from build123d import *

# Parameters (mm, degrees)
BOSS_EXTRUDE1_DEPTH = 8.89
SKETCH2_R           = 6.35
CUT_EXTRUDE1_DEPTH  = 27.197420728
SKETCH3_R           = 1.5
SKETCH3_R_2         = 1.45
BOSS_EXTRUDE2_DEPTH = 2.54


with BuildPart() as part:
    # Sketch1 → Boss-Extrude1 (new body)
    with BuildSketch(Plane.XY):
        with BuildLine():
            Line((-9.350252532, -14.130551756), (9.350252532, -14.130551756))
            Line((9.350252532, -14.130551756), (14.3, -9.180804288))
            Line((14.3, -9.180804288), (14.3, 12.34601478))
            ThreePointArc((14.3, 12.34601478), (0, 20.069448244), (-14.3, 12.34601478))
            Line((-14.3, 12.34601478), (-14.3, -9.180804288))
            Line((-14.3, -9.180804288), (-9.350252532, -14.130551756))
        make_face()
    extrude(amount=BOSS_EXTRUDE1_DEPTH)

    # Sketch2 → Cut-Extrude1 (cut, through all)
    with BuildSketch(Plane(origin=(0, 0, 0), x_dir=(-1, 0, 0), z_dir=(0, 0, -1))):
        with Locations((0, 5.99601478)):
            Circle(SKETCH2_R)
    extrude(amount=-CUT_EXTRUDE1_DEPTH, mode=Mode.SUBTRACT)

    # Sketch3 → Boss-Extrude2 (add)
    # profile 1 of 2: a face of its own
    with BuildSketch(Plane.XY.offset(8.89)):
        with BuildLine():
            Line((-14.3, 12.34601478), (-24.034198127, 9.287357095))
            ThreePointArc((-24.034198127, 9.287357095), (-26.45, 5.99601478), (-24.034198127, 2.704672465))
            Line((-24.034198127, 2.704672465), (-14.3, -0.35398522))
            Line((-14.3, -0.35398522), (-14.3, 12.34601478))
        make_face()
        with Locations((-16.2, 5.99601478)):
            Circle(SKETCH3_R, mode=Mode.SUBTRACT)
        with Locations((-23, 5.99601478)):
            Circle(SKETCH3_R_2, mode=Mode.SUBTRACT)
    # profile 2 of 2: a face of its own
    with BuildSketch(Plane.XY.offset(8.89)):
        with BuildLine():
            Line((14.3, 12.34601478), (14.3, -0.35398522))
            Line((14.3, -0.35398522), (24.034198127, 2.704672465))
            ThreePointArc((24.034198127, 2.704672465), (26.45, 5.99601478), (24.034198127, 9.287357095))
            Line((24.034198127, 9.287357095), (14.3, 12.34601478))
        make_face()
        with Locations((16.2, 5.99601478)):
            Circle(SKETCH3_R, mode=Mode.SUBTRACT)
        with Locations((23, 5.99601478)):
            Circle(SKETCH3_R_2, mode=Mode.SUBTRACT)
    extrude(amount=-BOSS_EXTRUDE2_DEPTH)


solid = part.part
Can you work these out from the model? Positions are in its coordinate system, mm. A direction names the side the tool comes from. Coordinates: 2 decimals unless noted, no trailing zeros. Loops run counter-clockwise (first coordinate to the right, second up) from the corner with the lowest first, then second, coordinate; pieces in that order, holes last. Notation, with made-up numbers: M 31.5,-39 L 83.5,-39 A21 cw 83.5,-11 Z; hole C 38.25,14.5 d9. An arc over 180 degrees is marked long. Return JSON: item names as keys, results as strings. Group by question number.
Item 1: Imagine slicing it at D-D (y = -1). Please give me the cut outline in (x, z), and give its area (3 significant figures).
Item 2: On a 3-axis mill with a long thin cutter (end or side, diameter ignored), from which of +Z, -Z, +X, -X, +Y, -Y can I reach the whole of each face in a straight line? I mean faces 1 (the flat face through (-14.3, 2, 3)), 2 (the flat face through (-19, 6, 6.35)), 3 (the flat face through (19, 6, 6.35)), 4 (the flat face through (14.3, 1, 3)). Say none if no direction works.
Item 3: Imagine slicing it at A-A (x = 0). Please give me the cut outline in (y, z).
Item 4: If I drill on L1, parallel to X at y = -2.5, z = 8.25; L2, parallel to Y at x = 23, z = 8.05; L3, parallel to Y at x = -16.2, z = 8, over which ranges is the centre line in solid material (lowest first)? Write a range as from..to.
Item 5: I'm going to push flat-ended pins straight in: pin 1 Ø4.5 at (x, y) = (23, 6) entering from +Z; pin 2 Ø6 at (x, y) = (21.5, 8.5) entering from -Z; pin 3 Ø1.5 at (y, z) = (8.5, 6) entering from -X; pin 4 Ø3 at (x, z) = (-16, 6.5) entering from -Y. Where does each tip first touch, or does it pass through?
Item 6: Imagine slicing it at B-B (z = 1.5). Please give me the cut outline in (x, y), and give its area (3 significant figures).
Item 7: Imagine slicing it at C-C (x = -23). Please give me the cut outline in (y, z).
Item 8: Thinking about a two-plate mould opening in X: for faces 5 (the cylindrical face through (-14.814, 5.422, 7.638)), 6 (the flat face through (0, -1, 0)), 7 (the flat face through (-19.24, 1.2, 7.64)), which applies, released by +X, released by -X, zero draft, split by the parting line, or undercut?
Verdict:
{
 "1": {"outline": "M -14.3,0 L 14.3,0 L 14.3,8.89 L -14.3,8.89 Z", "area": "254 mm^2"},
 "2": {"face 1": "-Z, -X, -Y", "face 2": "-Z, -X, +Y, -Y", "face 3": "-Z, +X, +Y, -Y", "face 4": "-Z, +X, -Y"},
 "3": {"outline": "M -14.13,0 L -0.35,0 L -0.35,8.89 L -14.13,8.89 Z; M 12.35,0 L 20.07,0 L 20.07,8.89 L 12.35,8.89 Z"},
 "4": {"L1": "x = -14.3..14.3", "L2": "y = 2.38..4.55, 7.45..9.61", "L3": "y = 0.24..4.5, 7.5..11.75"},
 "5": {"pin 1": "stops at z = 8.89", "pin 2": "stops at z = 6.35", "pin 3": "stops at x = -25.92", "pin 4": "stops at y = -0.29"},
 "6": {"outline": "M -14.3,-9.18 L -9.35,-14.13 L 9.35,-14.13 L 14.3,-9.18 L 14.3,12.35 A17.1 ccw -14.3,12.35 Z; hole C 0,6 d12.7", "area": "762 mm^2"},
 "7": {"outline": "M 2.38,6.35 L 4.55,6.35 L 4.55,8.89 L 2.38,8.89 Z; M 7.45,6.35 L 9.61,6.35 L 9.61,8.89 L 7.45,8.89 Z"},
 "8": {"face 5": "undercut", "face 6": "zero draft", "face 7": "released by -X"}
}
